Verification items for the finished model (mm, model axes). A direction names the side the tool comes from. Coordinates: 2 decimals unless noted, no trailing zeros. Loops run counter-clockwise (first coordinate to the right, second up) from the corner with the lowest first, then second, coordinate; pieces in that order, holes last.
Q1. Sectioned sample at C-C (y = 46). Enter the section's corners in (x, z).
Q2. Access from +Z, -Z, +X, -X, +Y, -Y to the whole of each face (thin tool, end or side, straight path). Record for faces 4 (the face through (29.868, 4.388, -79.064)), 5 (the face through (34.258, 11.993, 13.648)), 6 (the face through (69, 6, -66)).
Q3. Sectioned sample at A-A (z = -52). Enter the section's corners in (x, y), then the cut area to 3 significant figures.
Q4. Go/stop test with flat-tipped pins: P1, Ø7.5, axis at x = 92.5, y = 6, coming from the +Z side; P2, Ø12, axis at x = -1, y = 66, coming from the +Z side; P3, Ø6, axis at x = 0, z = 29, coming from the +Y side. Record where each tip stops, or that it passes through.
Q5. Material ranges on probe 1 along Z at (x, y) = (106, 4); probe 2 along Y at (x, z) = (-49, -27.5); probe 3 along X at (y, z) = (66, 0), recorded low to high.
Q6. Mould release check, pull along X, two halves, no side actions. Record for faces 1 (the face through (-51.02, 7.4, 5.04)), 2 (the face through (-9, 10, -9)), 3 (the face through (86, 7, -19.067)): +X half, -X half, draft (parallel to the pull), parting line (faces both ways), or undercut.
Q7. Sectioned sample at B-B (x = 30). Enter the section's corners in (y, z), then the cut area to 3 significant figures.
```python
from build123d import *

# Parameters (mm, degrees)
MAIN_BODY_DEPTH                 = 15
SKETCH3_R                       = 21.5
FRONT_EXTRUSION_DEPTH           = 67.3
SKETCH4_R                       = 10.1
SKETCH4_R_2                     = 13.5
SKETCH4_R_3                     = 2
SKETCH4_R_4                     = 1.7
SKETCH4_R_5                     = 3
BOLT_HOLES_DEPTH                = 162.060825691
BOLT_RECESSES_REAR_DEPTH        = 10
SKETCH6_R                       = 5.05
BOLT_RECESSES_FRONT_DEPTH       = 6.1
CUT_EXTRUDE1_START              = -32.2
SKETCH7_R                       = 21.5
SKETCH7_R_2                     = 20
CUT_EXTRUDE1_DEPTH              = 32.2
SKETCH8_R                       = 2.85
MOTOR_BOLT_HEAD_RECESSES_DEPTH  = 6
SKETCH9_R                       = 2
HEAT_SET_INSERT_HOLES_DEPTH     = 6
SKETCH10_R                      = 1.6
PCB_HEAT_SET_INSERT_HOLES_DEPTH = 4


with BuildPart() as part:
    # Sketch1 → Main Body (new body)
    with BuildSketch(Plane(origin=(0, 0, 0), x_dir=(1, 0, 0), z_dir=(0, 1, 0))):
        with BuildLine():
            Line((55, 84.067232452), (-55, 84.067232452))
            Line((-55, 84.067232452), (-100, 84.067232452))
            ThreePointArc((-100, 84.067232452), (-107.071067812, 81.138300264), (-110, 74.067232452))
            Line((-110, 74.067232452), (-110, 29.067232452))
            ThreePointArc((-110, 29.067232452), (-107.071067812, 21.99616464), (-100, 19.067232452))
            Line((-100, 19.067232452), (-72.737775696, 19.067232452))
            ThreePointArc((-72.737775696, 19.067232452), (-68.06426999, 17.90795326), (-64.474343867, 14.698901335))
            Line((-64.474343867, 14.698901335), (-37.18544323, -25.342509974))
            ThreePointArc((-37.18544323, -25.342509974), (0, -45), (37.18544323, -25.342509974))
            Line((37.18544323, -25.342509974), (64.474343867, 14.698901335))
            ThreePointArc((64.474343867, 14.698901335), (68.06426999, 17.90795326), (72.737775696, 19.067232452))
            Line((72.737775696, 19.067232452), (100, 19.067232452))
            ThreePointArc((100, 19.067232452), (107.071067812, 21.99616464), (110, 29.067232452))
            Line((110, 29.067232452), (110, 74.067232452))
            ThreePointArc((110, 74.067232452), (107.071067812, 81.138300264), (100, 84.067232452))
            Line((100, 84.067232452), (55, 84.067232452))
        make_face()
    extrude(amount=MAIN_BODY_DEPTH)

    # Sketch3 → Front Extrusion (add)
    with BuildSketch(Plane(origin=(0, 15, 0), x_dir=(1, 0, 0), z_dir=(0, 1, 0))):
        with Locations(Location((0, 0, 0), (0, 0, 270))):
            Circle(SKETCH3_R)
    extrude(amount=FRONT_EXTRUSION_DEPTH)

    # Sketch4 → Bolt Holes (cut, through all)
    with BuildSketch(Plane.XZ):
        with Locations(Location((0, 0, 0), (0, 0, 270))):
            Circle(SKETCH4_R)
        with Locations(Location((-55, -54.067232452, 0), (0, 0, 270))):
            Circle(SKETCH4_R_2)
        with Locations(Location((-10.677312396, 10.677312396, 0), (0, 0, 270))):
            Circle(SKETCH4_R_3)
        with Locations(Location((-10.677312396, -10.677312396, 0), (0, 0, 90))):
            Circle(SKETCH4_R_3)
        with Locations(Location((-69.142135624, -39.925096828, 0), (0, 0, 270))):
            Circle(SKETCH4_R_4)
        with Locations(Location((-69.142135624, -68.209368076, 0), (0, 0, 90))):
            Circle(SKETCH4_R_4)
        with Locations(Location((-40.857864376, -68.209368076, 0), (0, 0, 270))):
            Circle(SKETCH4_R_4)
        with Locations(Location((-40.857864376, -39.925096828, 0), (0, 0, 90))):
            Circle(SKETCH4_R_4)
        with Locations(Location((55, -54.067232452, 0), (0, 0, 90))):
            Circle(SKETCH4_R_2)
        with Locations(Location((69.142135624, -68.209368076, 0), (0, 0, 270))):
            Circle(SKETCH4_R_4)
        with Locations(Location((40.857864376, -68.209368076, 0), (0, 0, 90))):
            Circle(SKETCH4_R_4)
        with Locations(Location((40.857864376, -39.925096828, 0), (0, 0, 270))):
            Circle(SKETCH4_R_4)
        with Locations(Location((69.142135624, -39.925096828, 0), (0, 0, 90))):
            Circle(SKETCH4_R_4)
        with Locations(Location((10.677312396, -10.677312396, 0), (0, 0, 270))):
            Circle(SKETCH4_R_3)
        with Locations(Location((10.677312396, 10.677312396, 0), (0, 0, 90))):
            Circle(SKETCH4_R_3)
        with Locations(Location((-30, -76.067232452, 0), (0, 0, 270))):
            Circle(SKETCH4_R_5)
        with Locations(Location((-30, 10.932767548, 0), (0, 0, 270))):
            Circle(SKETCH4_R_5)
        with Locations(Location((30, -76.067232452, 0), (0, 0, 90))):
            Circle(SKETCH4_R_5)
        with Locations(Location((30, 10.932767548, 0), (0, 0, 90))):
            Circle(SKETCH4_R_5)
    extrude(amount=-BOLT_HOLES_DEPTH, mode=Mode.SUBTRACT)

    # Sketch5 → Bolt Recesses Rear (cut)
    with BuildSketch(Plane.XZ):
        with BuildLine():
            Line((-14.919953083, 6.434671709), (-9.987638511, 1.502357137))
            ThreePointArc((-9.987638511, 1.502357137), (-7.14177849, 7.14177849), (-1.502357137, 9.987638511))
            Line((-1.502357137, 9.987638511), (-6.434671709, 14.919953083))
            ThreePointArc((-6.434671709, 14.919953083), (-14.919953083, 14.919953083), (-14.919953083, 6.434671709))
        make_face()
        with BuildLine():
            Line((-14.919953083, -6.434671709), (-9.987638511, -1.502357137))
            ThreePointArc((-9.987638511, -1.502357137), (-7.14177849, -7.14177849), (-1.502357137, -9.987638511))
            Line((-1.502357137, -9.987638511), (-6.434671709, -14.919953083))
            ThreePointArc((-6.434671709, -14.919953083), (-14.919953083, -14.919953083), (-14.919953083, -6.434671709))
        make_face()
        with BuildLine():
            Line((6.434671709, -14.919953083), (1.502357137, -9.987638511))
            ThreePointArc((1.502357137, -9.987638511), (7.14177849, -7.14177849), (9.987638511, -1.502357137))
            Line((9.987638511, -1.502357137), (14.919953083, -6.434671709))
            ThreePointArc((14.919953083, -6.434671709), (14.919953083, -14.919953083), (6.434671709, -14.919953083))
        make_face()
        with BuildLine():
            Line((14.919953083, 6.434671709), (9.987638511, 1.502357137))
            ThreePointArc((9.987638511, 1.502357137), (7.14177849, 7.14177849), (1.502357137, 9.987638511))
            Line((1.502357137, 9.987638511), (6.434671709, 14.919953083))
            ThreePointArc((6.434671709, 14.919953083), (14.919953083, 14.919953083), (14.919953083, 6.434671709))
        make_face()
    extrude(amount=-BOLT_RECESSES_REAR_DEPTH, mode=Mode.SUBTRACT)

    # Sketch6 → Bolt Recesses Front (cut)
    with BuildSketch(Plane(origin=(0, 15, 0), x_dir=(1, 0, 0), z_dir=(0, 1, 0))):
        with Locations(Location((30, 76.067232452, 0), (0, 0, 270))):
            Circle(SKETCH6_R)
        with Locations(Location((-30, 76.067232452, 0), (0, 0, 270))):
            Circle(SKETCH6_R)
        with Locations(Location((-30, -10.932767548, 0), (0, 0, 270))):
            Circle(SKETCH6_R)
        with Locations(Location((30, -10.932767548, 0), (0, 0, 270))):
            Circle(SKETCH6_R)
    extrude(amount=-BOLT_RECESSES_FRONT_DEPTH, mode=Mode.SUBTRACT)

    # Sketch7 → Cut-Extrude1 (cut)
    with BuildSketch(Plane(origin=(0, 82.3, 0), x_dir=(1, 0, 0), z_dir=(0, 1, 0)).offset(CUT_EXTRUDE1_START)):
        with Locations(Location((0, 0, 0), (0, 0, 270))):
            Circle(SKETCH7_R)
        with Locations(Location((0, 0, 0), (0, 0, 270))):
            Circle(SKETCH7_R_2, mode=Mode.SUBTRACT)
    extrude(amount=CUT_EXTRUDE1_DEPTH, mode=Mode.SUBTRACT)

    # Sketch8 → Motor bolt head recesses (cut)
    with BuildSketch(Plane.XZ):
        with Locations(Location((-69.142135624, -39.925096828, 0), (0, 0, 270))):
            Circle(SKETCH8_R)
        with Locations(Location((-40.857864376, -39.925096828, 0), (0, 0, 270))):
            Circle(SKETCH8_R)
        with Locations(Location((-40.857864376, -68.209368076, 0), (0, 0, 270))):
            Circle(SKETCH8_R)
        with Locations(Location((-69.142135624, -68.209368076, 0), (0, 0, 270))):
            Circle(SKETCH8_R)
        with Locations(Location((40.857864376, -68.209368076, 0), (0, 0, 90))):
            Circle(SKETCH8_R)
        with Locations(Location((40.857864376, -39.925096828, 0), (0, 0, 90))):
            Circle(SKETCH8_R)
        with Locations(Location((69.142135624, -68.209368076, 0), (0, 0, 90))):
            Circle(SKETCH8_R)
        with Locations(Location((69.142135624, -39.925096828, 0), (0, 0, 90))):
            Circle(SKETCH8_R)
    extrude(amount=-MOTOR_BOLT_HEAD_RECESSES_DEPTH, mode=Mode.SUBTRACT)

    # Sketch9 → Heat-set insert holes (cut)
    with BuildSketch(Plane.XZ):
        with Locations(Location((-106, -74.067232452, 0), (0, 0, 270))):
            Circle(SKETCH9_R)
        with Locations(Location((-106, -32.067232452, 0), (0, 0, 270))):
            Circle(SKETCH9_R)
        with Locations(Location((-44, -32.067232452, 0), (0, 0, 270))):
            Circle(SKETCH9_R)
        with Locations(Location((-44, -74.067232452, 0), (0, 0, 270))):
            Circle(SKETCH9_R)
        with Locations(Location((44, -74.067232452, 0), (0, 0, 90))):
            Circle(SKETCH9_R)
        with Locations(Location((106, -74.067232452, 0), (0, 0, 90))):
            Circle(SKETCH9_R)
        with Locations(Location((44, -32.067232452, 0), (0, 0, 90))):
            Circle(SKETCH9_R)
        with Locations(Location((106, -32.067232452, 0), (0, 0, 90))):
            Circle(SKETCH9_R)
    extrude(amount=-HEAT_SET_INSERT_HOLES_DEPTH, mode=Mode.SUBTRACT)

    # Sketch10 → PCB Heat-set insert holes (cut)
    with BuildSketch(Plane.XZ):
        with Locations(Location((-95, -72.067232452, 0), (0, 0, 270))):
            Circle(SKETCH10_R)
        with Locations(Location((-95, -34.067232452, 0), (0, 0, 270))):
            Circle(SKETCH10_R)
        with Locations(Location((-55, -34.067232452, 0), (0, 0, 270))):
            Circle(SKETCH10_R)
        with Locations(Location((-55, -72.067232452, 0), (0, 0, 270))):
            Circle(SKETCH10_R)
        with Locations(Location((95, -72.067232452, 0), (0, 0, 90))):
            Circle(SKETCH10_R)
        with Locations(Location((55, -72.067232452, 0), (0, 0, 90))):
            Circle(SKETCH10_R)
        with Locations(Location((55, -34.067232452, 0), (0, 0, 90))):
            Circle(SKETCH10_R)
        with Locations(Location((95, -34.067232452, 0), (0, 0, 90))):
            Circle(SKETCH10_R)
    extrude(amount=-PCB_HEAT_SET_INSERT_HOLES_DEPTH, mode=Mode.SUBTRACT)


solid = part.part
```
Geometry check:
1. outline: circle Ø43 at (0, 0); hole circle Ø4 at (-10.68, -10.68); hole circle Ø4 at (-10.68, 10.68); hole circle Ø20.2 at (0, 0); hole circle Ø4 at (10.68, -10.68); hole circle Ø4 at (10.68, 10.68)
2. face 4: +Y, -Y
2. face 5: +Y
2. face 6: -Y
3. outline: (-110, 0) - (-68.34, 0) - (-68.34, 15) - (-110, 15) - close; (-41.66, 0) - (41.66, 0) - (41.66, 15) - (-41.66, 15) - close; (68.34, 0) - (110, 0) - (110, 15) - (68.34, 15) - close
3. area: 2,500 mm2
4. P1: stops at z = -19.07
4. P2: stops at z = 20
4. P3: stops at y = 15
5. probe 1: z = -82.07 to -76.07, -72.07 to -34.07, -30.07 to -21.07
5. probe 2: y = 0 to 15
5. probe 3: x = -20 to -10.1, 10.1 to 20
6. face 1: -X half
6. face 2: undercut
6. face 3: draft
7. outline: (0, -84.07) - (15, -84.07) - (15, -81.12) - (8.9, -81.12) - (8.9, -79.07) - (0, -79.07) - close; (0, -73.07) - (8.9, -73.07) - (8.9, -71.02) - (15, -71.02) - (15, 5.88) - (8.9, 5.88) - (8.9, 7.93) - (0, 7.93) - close; (0, 13.93) - (8.9, 13.93) - (8.9, 15.98) - (15, 15.98) - (15, 33.54) - (0, 33.54) - close
7. area: 1,530 mm2
